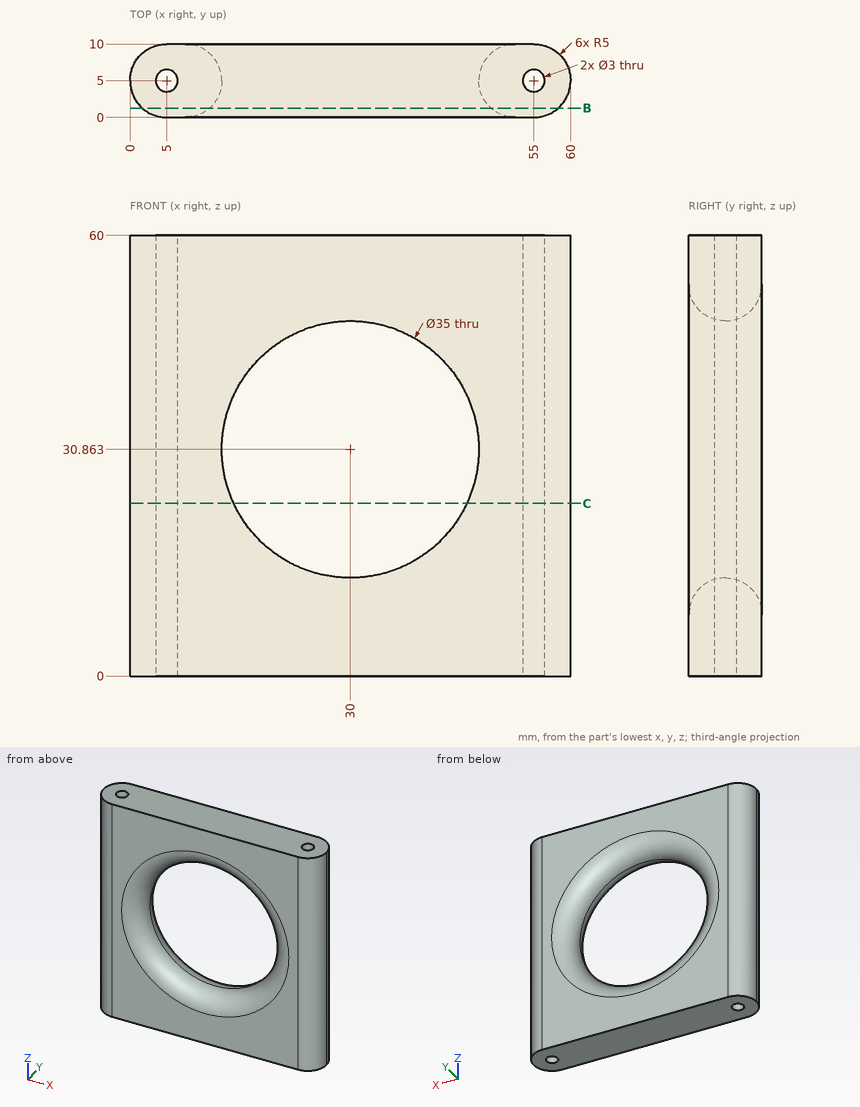
Input: dimensioned drawing with shaded views. Units: mm. Origin: part minimum x, y, z. Give positions to 0.01 mm unless a question says otherwise; leave off trailing zeros. Write each loop counter-clockwise with the first axis right and the second up, starting at its lowest first coordinate (ties: lowest second). Pieces come first, ordered by that corner, then holes. Notation, with made-up numbers: (-31, 74.25) -> (20, 74.25) arc R22 cw to (20, 96.25) -> close; hole circle Ø11 at (-33.5, 27.25). An arc over 180 degrees is marked (long way). Answer as a JSON object with one key per item and string values.
1. Contact query for flat-ended pins moving along their axis: pin 1 (5 mm diameter, centred on x = 37, z = 14.5, fed in from -Y); pin 2 (1.5 mm diameter, centred on y = 7.5, z = 21, fed in from -X). Output: stop coordinate, or through.
Ans:
{"pin 1": "stops at y = 0.51", "pin 2": "stops at x = 0.32"}
2. Cut plane C-C on z = 23.5. Count the separate pieces of the cut face and the enclosed holes in it.
Ans:
{"separate pieces": "2", "enclosed holes": "2"}
3. Cut plane B-B on y = 1.25. Output: boundary loops of the cut face in (x, z) (1 decimal), and give its area (3 significant figures).
Ans:
{"outline": "(1.7, 0) -> (58.3, 0) -> (58.3, 60) -> (1.7, 60) -> close; hole circle Ø38.4 at (30, 30.9)", "area": "2,240 mm^2"}
4. Ray query, probe 1 along Y at (x, z) = (55, 30); probe 2 along X at (y, z) = (4.75, 46) (1 decimal); probe 3 along X at (y, z) = (6, 43). Return the intervals inside material, ascending. Write a range as from..to.
Ans:
{"probe 1": "y = 0..3.5, 6.5..10", "probe 2": "x = 0..3.5, 6.5..21.2, 38.8..53.5, 56.5..60", "probe 3": "x = 0.1..3.88, 6.12..17.25, 42.75..53.88, 56.12..59.9"}
